Job drawing, mm, ordinate dimensions from the low corner. One solid piece. A direction names the side the tool comes from. Give positions to 0.01 mm unless a question says otherwise; leave off trailing zeros. Loops run counter-clockwise (first coordinate to the right, second up) from the corner with the lowest first, then second, coordinate; pieces in that order, holes last. Notation, with made-up numbers: M 59.25,32 L 73.25,32 A17 cw 73.25,48 Z; hole C 81.25,23.5 d7. An arc over 180 degrees is marked long. Answer in a Markdown table with one row per item.
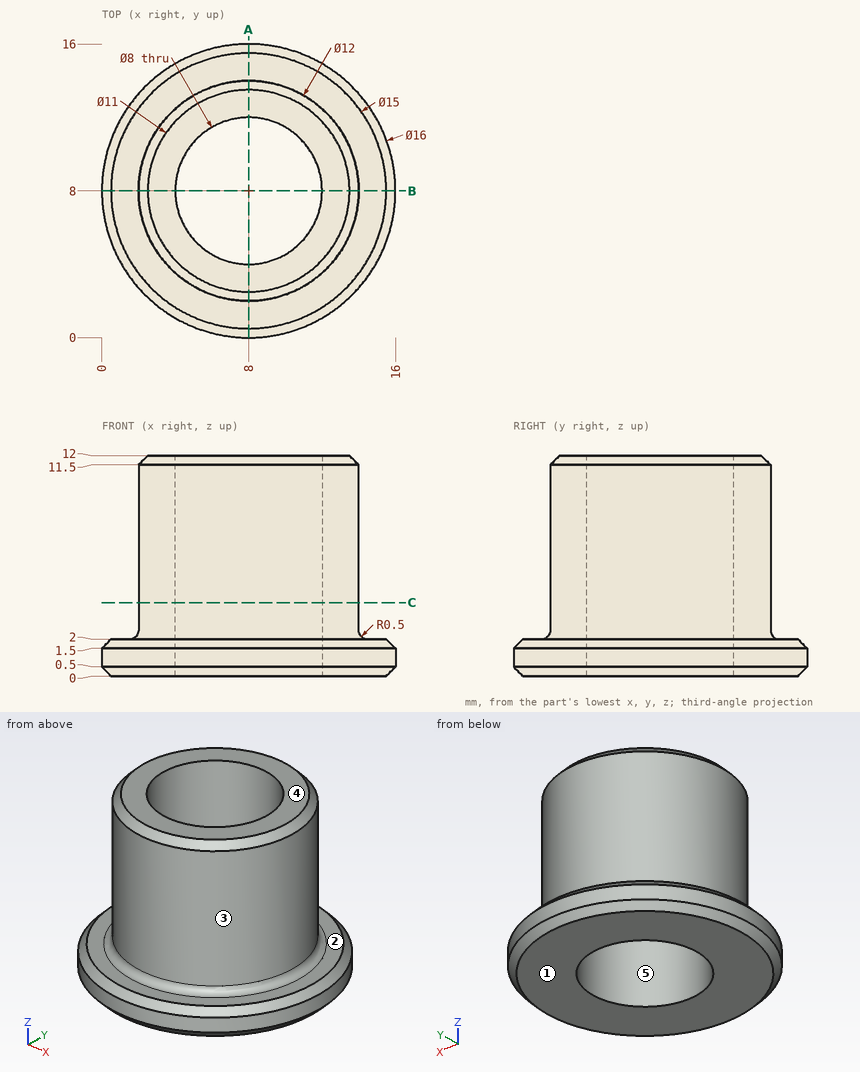
(1) Drill centre lines: line 1 along Y through (x, z) = (8, 5); line 2 along Y through (x, z) = (9.75, 7); line 3 along X through (y, z) = (6.5, 5). Where is each one in solid material? Low to high.
Recorded:
| item | result |
|---|---|
| line 1 | y = 2 to 4, 12 to 14 |
| line 2 | y = 2.26 to 4.4, 11.6 to 13.74 |
| line 3 | x = 2.19 to 4.29, 11.71 to 13.81 |
(2) Pin check, flat tips, straight feed: pin 1 Ø2 at (x, z) = (9.5, 6.5) entering from +Y; pin 2 Ø1 at (y, z) = (10.5, 8) entering from +X; pin 3 Ø1.5 at (x, z) = (6, 5.5) entering from -Y. Stop position of each tip, or through.
Recorded:
| item | result |
|---|---|
| pin 1 | stops at y = 13.98 |
| pin 2 | stops at x = 13.66 |
| pin 3 | stops at y = 2.13 |
(3) Saw through at C-C (z = 4). Write the cut outline in (x, y), plus the area to 3 significant figures.
Recorded:
| item | result |
|---|---|
| outline | C 8,8 d12; hole C 8,8 d8 |
| area | 62.8 mm^2 |
(4) Pull direction Y, two halves, no side cores. Call the marked faces 3, 4 and 5: +Y half, -Y half, draft (parallel to the pull), parting line (faces both ways), or undercut.
Recorded:
| item | result |
|---|---|
| face 3 | parting line |
| face 4 | draft |
| face 5 | undercut |
(5) Saw through at A-A (x = 8). Write the cut outline in (y, z), plus the area to 3 significant figures.
Recorded:
| item | result |
|---|---|
| outline | M 0,0.5 L 0.5,0 L 4,0 L 4,12 L 2.5,12 L 2,11.5 L 2,2.5 A0.5 cw 1.5,2 L 0.5,2 L 0,1.5 Z; M 12,0 L 15.5,0 L 16,0.5 L 16,1.5 L 15.5,2 L 14.5,2 A0.5 cw 14,2.5 L 14,11.5 L 13.5,12 L 12,12 Z |
| area | 55.4 mm^2 |
(6) Which spindle directions (+Z, -Z, +X, -X, +Y, -Y) get a long thin tool onto all of the face, cutting with end or side? Do the marked faces 1 and 2. Say none if no direction does.
Recorded:
| item | result |
|---|---|
| face 1 | -Z, +X, -X, +Y, -Y |
| face 2 | +Z |
